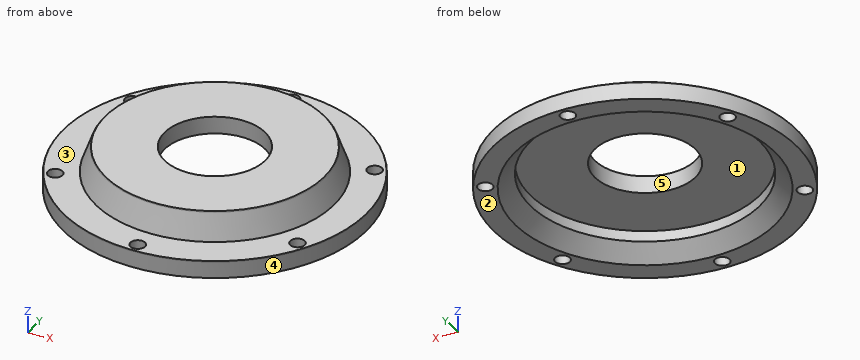
from build123d import *
from OCP.BRepFilletAPI import BRepFilletAPI_MakeChamfer

# Parameters (mm, degrees)
SKETCH1_R            = 35
BOSS_EXTRUDE1_DEPTH  = 10
SKETCH2_R            = 26.5
CUT_EXTRUDE1_DEPTH   = 6
CHAMFER1_SIZE        = 3.5
SKETCH5_R            = 35
SKETCH5_R_2          = 27.5
CUT_EXTRUDE3_DEPTH   = 6
CHAMFER3_SIZE        = 6
CHAMFER3_SIZE_2      = 2.183821406
SKETCH6_R            = 11.625
CUT_EXTRUDE4_DEPTH   = 6
M3_CLEARANCE_HOLE1_D = 3.4
CIRPATTERN1_COUNT    = 6
CHAMFER4_SIZE        = 0.2
CHAMFER4_SIZE2       = 0.072794047
CHAMFER4_SIZE2_2     = 0.089295118


with BuildPart() as part:
    # Sketch1 → Boss-Extrude1 (new body)
    with BuildSketch(Plane.XY):
        Circle(SKETCH1_R)
    extrude(amount=-BOSS_EXTRUDE1_DEPTH)

    # Sketch2 → Cut-Extrude1 (cut)
    with BuildSketch(Plane(origin=(0, 0, -10), x_dir=(-1, 0, 0), z_dir=(0, 0, -1))):
        Circle(SKETCH2_R)
    extrude(amount=-CUT_EXTRUDE1_DEPTH, mode=Mode.SUBTRACT)

    # Chamfer1
    chamfer1_edges = [part.edges().sort_by_distance(p)[0] for p in [
        (26.5, 0, -10),
    ]]
    chamfer(chamfer1_edges, length=CHAMFER1_SIZE)

    # Sketch5 → Cut-Extrude3 (cut)
    with BuildSketch(Plane.XY):
        Circle(SKETCH5_R)
        Circle(SKETCH5_R_2, mode=Mode.SUBTRACT)
    extrude(amount=-CUT_EXTRUDE3_DEPTH, mode=Mode.SUBTRACT)

    # Chamfer3
    # the kernel refuses this chamfer: 6, 2.183821406 mm, written as the material it takes off along each edge
    with BuildSketch(Plane(origin=(0, 0, 0), x_dir=(1, 0, 0), z_dir=(0, -1, 0))) as chamfer3_piece_1_section:
        Polygon((27.5, -CHAMFER3_SIZE), (27.5 - CHAMFER3_SIZE_2, 0), (27.5, 0), align=None)
    chamfer3_piece_1 = revolve(axis=Axis((0, 0, 0), (0, 0, 1)), mode=Mode.PRIVATE)
    chamfer3_piece_1 = split(chamfer3_piece_1, bisect_by=Plane(origin=(-26.469518779, 0, -6), z_dir=(0, 0, 1)), keep=Keep.TOP, mode=Mode.PRIVATE)
    add(chamfer3_piece_1, mode=Mode.SUBTRACT)

    # Sketch6 → Cut-Extrude4 (cut)
    with BuildSketch(Plane.XY):
        Circle(SKETCH6_R)
    extrude(amount=-CUT_EXTRUDE4_DEPTH, mode=Mode.SUBTRACT)

    # M3 Clearance Hole1 (through all)
    with Locations(Plane(origin=(0, 32.5, -6), x_dir=(1, 0, 0), z_dir=(0, 0, 1))):
        with Locations((0, 0)):
            m3_clearance_hole1 = Hole(M3_CLEARANCE_HOLE1_D / 2)

    # CirPattern1: M3 Clearance Hole1 ×6 about axis
    cirpattern1_axis = Axis((0, 0, 0), (0, 0, 1))
    for i in range(1, CIRPATTERN1_COUNT):
        add(m3_clearance_hole1.rotate(cirpattern1_axis, i * 360 / CIRPATTERN1_COUNT), mode=Mode.SUBTRACT)

    # Chamfer4: one chamfer whose edges measure the first distance from different faces: ONE call of the kernel's chamfer builder (chamfer() names one face for all edges)
    chamfer4_edges_1 = [part.edges().sort_by_distance(p)[0] for p in [
        (-35, 0, -6),
    ]]
    chamfer4_side_1 = [part.faces().sort_by_distance(p)[0] for p in [
        (-35, 0, -8),
    ]]
    chamfer4_edges_2 = [part.edges().sort_by_distance(p)[0] for p in [
        (-25.316178594, 0, 0),
    ]]
    chamfer4_side_2 = [part.faces().sort_by_distance(p)[0] for p in [
        (-26.408089297, 0, -3),
    ]]
    chamfer4 = BRepFilletAPI_MakeChamfer(part.part.solid().wrapped)
    for e in chamfer4_edges_1:
        chamfer4.Add(CHAMFER4_SIZE, CHAMFER4_SIZE2, e.wrapped, chamfer4_side_1[0].wrapped)  # the first distance lies on this face
    for e in chamfer4_edges_2:
        chamfer4.Add(CHAMFER4_SIZE, CHAMFER4_SIZE2_2, e.wrapped, chamfer4_side_2[0].wrapped)  # the first distance lies on this face
    add(Compound.cast(chamfer4.Shape()), mode=Mode.REPLACE)


solid = part.part
Work out the finished part from the listing and answer in its coordinate system (mm). Face numbers are marked on the shaded views. A direction names the side the tool comes from. Round coordinates to 2 decimals unless told otherwise and drop trailing zeros. Loops run counter-clockwise (first coordinate to the right, second up) from the corner with the lowest first, then second, coordinate; pieces in that order, holes last. Notation, with made-up numbers: M 87,30 L 96,30 A13 cw 96,44 Z; hole C 43,58 d3. An arc over 180 degrees is marked long. One line per question, with ' | ' between items. Start each with the question number.
(1) Find the intervals of material crossed by line 1 (Y direction, x = 0, z = -9.1); line 2 (Z direction, x = 8.5, y = 11); line 3 (Y direction, x = 0, z = -1.1) (3 decimals), in increasing order.
(2) A cutting plane is placed at A-A on y = 0. Write down the section's boundary in (x, z) (3 decimals), plus the area to 3 significant figures.
(3) For a pull along Y with two mould halves and no side action, classify the marked faces 3, 4 and 5 as released by +Y, released by -Y, zero draft, split by the parting line, or undercut.
(4) A tool of negligible diameter and unlimited length cuts with its end or side. For the marked faces 1 and 2, from which of +Z, -Z, +X, -X, +Y, -Y can it reach the whole face along a straight path? Write none if from no direction.
(5) Flat-ended cylindrical pins translate along their axes: pin 1 Ø4.5 at (x, y) = (28.15, 16.25) entering from +Z; pin 2 Ø6 at (x, z) = (20, -6.5) entering from +Y; pin 3 Ø6 at (x, y) = (-4, 5) entering from -Z; pin 4 Ø1.5 at (x, z) = (4, -4.5) entering from +Y. Find the tip coordinate at first contact, or state that the pin passes through.
(6) A cutting plane is placed at C-C on z = -8. Write down the section's boundary in (x, y), plus the area to 3 significant figures.
(7) A cutting plane is placed at B-B on x = 0. Give the number of separate pieces and of enclosed holes in the cut face, plus the area to 3 significant figures.
Geometry check:
1) line 1: y = -35 to -34.2, -30.8 to -29.1, 29.1 to 30.8, 34.2 to 35 | line 2: z = -4 to 0 | line 3: y = -25.717 to -11.625, 11.625 to 25.717
2) outline: M -35,-10 L -30,-10 L -26.5,-6.5 L -26.5,-4 L -11.625,-4 L -11.625,0 L -25.227,0 L -25.385,-0.188 L -27.5,-6 L -34.927,-6 L -35,-6.2 Z; M 11.625,-4 L 26.5,-4 L 26.5,-6.5 L 30,-10 L 35,-10 L 35,-6.2 L 34.927,-6 L 27.5,-6 L 25.385,-0.188 L 25.227,0 L 11.625,0 Z | area: 174 mm²
3) face 3: zero draft | face 4: split by the parting line | face 5: undercut
4) face 1: -Z | face 2: -Z, +X, -X, +Y, -Y
5) pin 1: stops at z = -6 | pin 2: stops at y = 30.59 | pin 3: passes through | pin 4: stops at y = 26.95
6) outline: C 0,0 d70; hole C -28.15,-16.25 d3.4; hole C -28.15,16.25 d3.4; hole C 0,0 d56; hole C 0,-32.5 d3.4; hole C 0,32.5 d3.4; hole C 28.15,-16.25 d3.4; hole C 28.15,16.25 d3.4 | area: 1,330 mm²
7) separate pieces: 4 | enclosed holes: 0 | area: 146 mm²
